Build history of the part. All positions in model axes, mm. Face numbers are marked on the shaded views. A direction names the side the tool comes from. Round coordinates to 2 decimals unless told otherwise and drop trailing zeros. Loops run counter-clockwise (first coordinate to the right, second up) from the corner with the lowest first, then second, coordinate; pieces in that order, holes last.
from build123d import *

# Parameters (mm, degrees)
SKETCH1_W               = 22.225
SKETCH1_H               = 22.225
BOSS_EXTRUDE1_DEPTH     = 30
SKETCH3_W               = 25.4
SKETCH3_H               = 25.4
BOSS_EXTRUDE2_DEPTH     = 3
BOSS_EXTRUDE3_DEPTH     = 25.4
BOSS_EXTRUDE4_DEPTH     = 19.43
CUT_EXTRUDE1_DEPTH      = 75.504751526
CUT_EXTRUDE1_DEPTH_BACK = 75.504751526
SKETCH5_R               = 3.175
CUT_EXTRUDE2_DEPTH      = 4.38
CHAMFER1_SIZE           = 2


with BuildPart() as part:
    # Sketch1 → Boss-Extrude1 (new body)
    with BuildSketch(Plane.XY):
        Rectangle(SKETCH1_W, SKETCH1_H)
    extrude(amount=BOSS_EXTRUDE1_DEPTH)

    # Sketch3 → Boss-Extrude2 (add)
    with BuildSketch(Plane.XY.offset(30)):
        Rectangle(SKETCH3_W, SKETCH3_H)
    extrude(amount=BOSS_EXTRUDE2_DEPTH)

    # Sketch4 → Boss-Extrude3 (add)
    with BuildSketch(Plane(origin=(0, 12.7, 0), x_dir=(1, 0, 0), z_dir=(0, 1, 0))):
        Polygon((-12.725, -33), (-12.725, -68.34), (-9.725, -68.34), (-9.725, -55.45), (-6.725, -55.45), (-6.725, -52.45), (-9.725, -52.45), (-9.725, -33), align=None)
        Polygon((9.725, -33), (12.725, -33), (12.725, -68.34), (9.725, -68.34), (9.725, -55.45), (6.725, -55.45), (6.725, -52.45), (9.725, -52.45), align=None)
    extrude(amount=-BOSS_EXTRUDE3_DEPTH)

    # Sketch6 → Boss-Extrude4 (add)
    with BuildSketch(Plane.XY.offset(68.34)):
        Polygon((-12.725, -12.7), (-17.095, -7.555), (-17.095, 7.555), (-12.725, 12.7), align=None)
    extrude(amount=-BOSS_EXTRUDE4_DEPTH)

    # Sketch5 → Cut-Extrude1 (cut, two sides: drawn at the far end of the back side and taken through both)
    with BuildSketch(Plane.ZY.offset(-9.725).offset(-CUT_EXTRUDE1_DEPTH_BACK)):
        with Locations((58.625, 0)):
            Circle(SKETCH5_R)
    extrude(amount=CUT_EXTRUDE1_DEPTH + CUT_EXTRUDE1_DEPTH_BACK, mode=Mode.SUBTRACT)

    # Sketch7 → Cut-Extrude2 (cut)
    with BuildSketch(Plane.ZY.offset(17.095)):
        Polygon((61.976518313, 5.805), (55.273481687, 5.805), (51.921963375, 0), (55.273481687, -5.805), (61.976518313, -5.805), (65.328036625, 0), align=None)
    extrude(amount=-CUT_EXTRUDE2_DEPTH, mode=Mode.SUBTRACT)

    # Chamfer1
    chamfer1_edges = [part.edges().sort_by_distance(p)[0] for p in [
        (11.1125, -11.1125, 15),
        (-11.1125, -11.1125, 15),
        (-11.1125, 11.1125, 15),
        (11.1125, 11.1125, 15),
    ]]
    chamfer(chamfer1_edges, length=CHAMFER1_SIZE)


solid = part.part
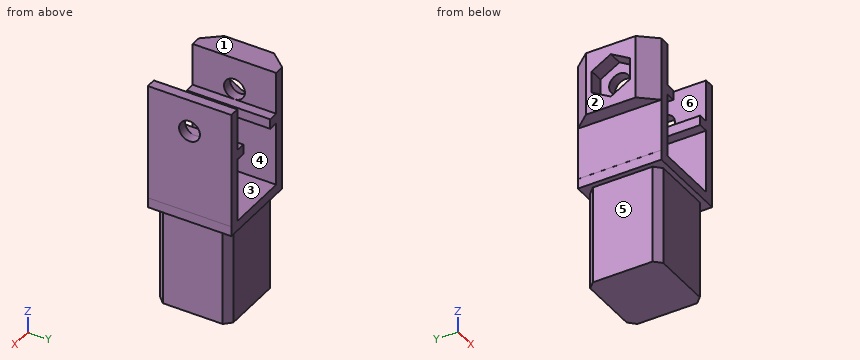
(1) Slice it at C-C on z = 14.5. List the corners of the cut face in (x, y).
Responses:
outline: (-11.11, -9.11) - (-9.11, -11.11) - (9.11, -11.11) - (11.11, -9.11) - (11.11, 9.11) - (9.11, 11.11) - (-9.11, 11.11) - (-11.11, 9.11) - close
(2) Slice it at D-D on y = -1.75. Count the separate pieces of the cut face and the enclosed holes in it, plus the area to 3 significant figures.
Responses:
separate pieces: 3
enclosed holes: 0
area: 976 mm2
(3) Slice it at B-B on x = -3. List the corners of the cut face in (y, z), plus the area to 3 significant figures.
Responses:
outline: (-12.7, 30) - (-11.11, 30) - (-11.11, 0) - (11.11, 0) - (11.11, 30) - (12.7, 30) - (12.7, 33) - (-12.7, 33) - close
area: 743 mm2
(4) Pull direction X, two halves, no side cores. Call the marked faces 1, 2 and 3: +X half, -X half, draft (parallel to the pull), parting line (faces both ways), or undercut.
Responses:
face 1: draft
face 2: -X half
face 3: undercut
(5) Which spindle directions (+Z, -Z, +X, -X, +Y, -Y) get a long thin tool onto all of the face, cutting with end or side? Do the marked faces 4, 5 and 6. Say none if no direction does.
Responses:
face 4: +Y, -Y
face 5: -Z, -X, +Y, -Y
face 6: +Z, +Y, -Y
(6) Slice it at A-A on z = 39.5. List the corners of the cut face in (x, y) (3 decimals), plus the area to 3 significant figures.
Responses:
outline: (-12.725, -12.7) - (-9.725, -12.7) - (-9.725, 12.7) - (-12.725, 12.7) - close; (9.725, -12.7) - (12.725, -12.7) - (12.725, 12.7) - (9.725, 12.7) - close
area: 152 mm2
(7) Pin check, flat tips, straight feed: P1, Ø1, axis at y = -8.5, z = 11.5, coming from the -X side; P2, Ø12.5, axis at y = 4, z = 38, coming from the -X side (3 decimals); P3, Ø8, axis at x = -4, y = -7, coming from the +Z side. Stop position of each tip, or through.
Responses:
P1: stops at x = -11.11
P2: stops at x = -12.725
P3: stops at z = 55.45
(8) Probe line 1 (Z direction, x = 10.6, y = 0); line 2 (Z direction, x = -7.5, y = 11.75); line 3 (X direction, y = 1.5, z = 54) (3 decimals). List the from-to ranges inside material, lowest first.
Responses:
line 1: z = 0 to 55.45, 61.8 to 68.34
line 2: z = 30 to 33, 52.45 to 55.45
line 3: x = -12.715 to -6.725, 6.725 to 12.725
